Autodesk Inventor part; units mm, degrees
ref_plane "YZ Plane" through (0, 0, 0) normal (1, 0, 0) x (0, 1, 0)
ref_plane "XZ Plane" through (0, 0, 0) normal (0, 1, 0) x (-1, 0, 0)
ref_plane "XY Plane" through (0, 0, 0) normal (0, 0, 1) x (1, 0, 0)
sketch "Sketch1" plane through (0, 0, 0) normal (0, 0, 1) x (1, 0, 0)
  circle A0 centre (43.3303, -43.3303) radius 1.5
  circle A1 centre (32.0698, -32.0698) radius 1.5
  arc A2 (2.3181, 4.753) -> (-4.753, -2.3181) centre (-1.2174, 1.2174) ccw
  line L0 (-4.753, -2.3181) -> (44.7445, -51.8156)
  line L1 (44.7445, -51.8156) -> (51.8156, -44.7445)
  line L2 (51.8156, -44.7445) -> (2.3181, 4.753)
  line L3 (44.7445, -51.8156) -> (34.845, -41.9161)
  line L4 (44.7445, -51.8156) -> (51.8156, -44.7445)
  line L5 (51.8156, -44.7445) -> (41.9161, -34.845)
  line L6 (34.845, -41.9161) -> (41.9161, -34.845)
  line L7 (44.7445, -51.8156) -> (42.6232, -53.9369)
  line L8 (42.6232, -53.9369) -> (32.7237, -44.0374)
  line L9 (32.7237, -44.0374) -> (34.845, -41.9161)
  line L10 (51.8156, -44.7445) -> (53.9369, -42.6232)
  line L11 (53.9369, -42.6232) -> (44.0374, -32.7237)
  line L12 (44.0374, -32.7237) -> (41.9161, -34.845)
  line L13 (44.391, -52.1691) -> (34.4915, -42.2697)
  line L14 (52.1691, -44.391) -> (42.2697, -34.4915)
  point P0 (0, 0)
  dimension "d1" = 7
  dimension "d2" = 3
  dimension "d3" = 3
  dimension "d10" = 0.5
  dimension "d11" = 0.5
extrude "Extrusion1" add sketch "Sketch1" along normal blind 2.5 contours L12 L14 L10 L2 | L2 L1 L0 L6 | L0 L7 L13 L9 | L12 L11 L10 L14 | L13 L7 L8 L9
sketch "Sketch2" plane through (0, 0, 0) normal (0, 0, -1) x (-1, 0, 0)
  line L0 (-32.7237, -44.0374) -> (-42.6232, -53.9369)
  line L1 (4.753, -2.3181) -> (-44.7445, -51.8156)
  line L2 (-42.6232, -53.9369) -> (-44.7445, -51.8156)
  line L3 (-44.0374, -32.7237) -> (-32.7237, -44.0374)
  line L4 (-53.9369, -42.6232) -> (-44.0374, -32.7237)
  line L5 (-51.8156, -44.7445) -> (-2.3181, 4.753)
  line L6 (-51.8156, -44.7445) -> (-53.9369, -42.6232)
  line L7 (-32.7237, -44.0374) -> (-34.845, -41.9161)
  line L8 (-44.0374, -32.7237) -> (-32.7237, -44.0374)
  line L9 (-44.0374, -32.7237) -> (-41.9161, -34.845)
  line L10 (-34.6683, -42.0929) -> (-44.5677, -51.9924)
  line L11 (-42.0929, -34.6683) -> (-51.9924, -44.5677)
  point P0 (0, 0)
  dimension "d12" = 0.25
  dimension "d13" = 0.25
extrude "Extrusion2" add sketch "Sketch2" along normal blind 3 contours L0 L2 L10 L3 | L11 L6 L4 L3
sketch "Sketch3" plane through (0, 0, 2.5) normal (0, 0, 1) x (1, 0, 0)
  line L0 (-4.753, -2.3181) -> (44.7445, -51.8156)
  line L1 (42.6232, -53.9369) -> (44.7445, -51.8156)
  line L2 (32.7237, -44.0374) -> (42.6232, -53.9369)
  line L3 (53.9369, -42.6232) -> (44.0374, -32.7237)
  line L4 (51.8156, -44.7445) -> (53.9369, -42.6232)
  line L5 (51.8156, -44.7445) -> (2.3181, 4.753)
  line L6 (41.9161, -34.845) -> (44.0374, -32.7237)
  line L7 (51.9924, -44.5677) -> (42.0929, -34.6683)
  line L8 (34.6683, -42.0929) -> (44.5677, -51.9924)
  line L9 (34.6683, -42.0929) -> (32.7237, -44.0374)
  line L10 (44.0374, -32.7237) -> (32.7237, -44.0374)
  point P0 (0, 0)
extrude "Extrusion3" add sketch "Sketch3" along normal blind 6 contours L8 L1 L2 L9 | L6 L3 L4 L7
properties part number "eye_cam_arm_brace"
Design review of the part built by this model. Coordinates are the model's own, in mm. A direction names the side the tool comes from. Give positions to 0.01 mm unless a question says otherwise; leave off trailing zeros. Loops run counter-clockwise (first coordinate to the right, second up) from the corner with the lowest first, then second, coordinate; pieces in that order, holes last. Notation, with made-up numbers: (70.5, -26) -> (83.5, -26) arc R25 cw to (83.5, 2) -> close; hole circle Ø1 at (21, 42). An arc over 180 degrees is marked (long way). One line per question, with ' | ' between items. Start each with the question number.
(1) Draft analysis for pull direction X (two halves, no side actions). For faces 4 (the face through (45, -43, 0)), 5 (the face through (48, -39, -3)), 6 (the face through (37.743, -49.056, 2.67)), state which applies: +X half, -X half, draft (parallel to the pull), parting line (faces both ways), or undercut.
(2) We need section C-C (x = 37.25). State the section outline as (y, z) points, and give its area (3 significant figures).
(3) We need section D-D (z = 1.75). State the section outline as (x, y) points, and give its area (3 significant figures).
(4) For faces 1 (the face through (46.973, -39.549, -1.479)), 2 (the face through (39, -48, -3)), 3 (the face through (47.112, -39.687, 5.458)), list the 3-axis set-ups (+Z, -Z, +X, -X, +Y, -Y) from which the entire face can be reached by the end or side of a thin tool; tool diameter is ignored.
(5) We need section A-A (z = 5.25). State the section outline as (x, y) points, and give its area (3 significant figures).
(6) Insertion check: P1, Ø1, axis at x = 44, z = 2, coming from the +Y side; P2, Ø6, axis at y = -37.5, z = 6, coming from the -X side; P3, Ø8, axis at x = 44, y = -45, coming from the -Z side; P4, Ø2.5, axis at x = 43.33, y = -43.33, coming from the +Z side. Each pin has a flat end and moves straight along its axis. Give the tip position at first contact, or say it passes through.
(7) We need section B-B (y = -47). State the section outline as (x, z) points.
(8) For line 1 (Z direction, x = 41.25, y = -48); line 2 (X direction, y = -43.5, z = -0.75); line 3 (Y direction, x = 43.5, z = -2.5), list the stretches that pass through material, from the lowest coordinate up.
The answers:
1) face 4: undercut | face 5: draft | face 6: -X half
2) outline: (-48.56, -3) -> (-44.67, -3) -> (-44.67, 0) -> (-39.51, 0) -> (-39.51, 2.5) -> (-44.67, 2.5) -> (-44.67, 8.5) -> (-48.56, 8.5) -> close | area: 57.6 mm^2
3) outline: (32.72, -44.04) -> (42.62, -53.94) -> (53.94, -42.62) -> (44.04, -32.72) -> close; hole circle Ø3 at (43.33, -43.33) | area: 217 mm^2
4) face 1: -Z | face 2: -Z, +X, -X, +Y, -Y | face 3: +Z
5) outline: (32.72, -44.04) -> (42.62, -53.94) -> (44.57, -51.99) -> (34.67, -42.09) -> close; (42.09, -34.67) -> (51.99, -44.57) -> (53.94, -42.62) -> (44.04, -32.72) -> close | area: 77.0 mm^2
6) P1: stops at y = -32.72 | P2: stops at x = 42.09 | P3: stops at z = 0 | P4: passes through
7) outline: (35.69, -3) -> (39.58, -3) -> (39.58, 0) -> (49.56, 0) -> (49.56, 2.5) -> (39.58, 2.5) -> (39.58, 8.5) -> (35.69, 8.5) -> close
8) line 1: z = 0 to 2.5 | line 2: x = 33.26 to 36.08, 50.92 to 53.06 | line 3: y = -53.06 to -50.92, -36.08 to -33.26
